CAD build for the part. Positions are in the model's coordinates, mm. A direction names the side the tool comes from. Coordinates: 2 decimals unless noted, no trailing zeros. Order: outer loops, then holes, each group sorted by start corner. A loop starts at its lowest first (then second) coordinate and runs counter-clockwise, first axis right, second up. Notation, with made-up numbers: (-32, -34.75) - (-9, -34.75) arc R26 ccw to (-9, 2.25) - close; hole circle Ø4 at (-8.75, -36.5). An arc over 180 degrees is marked (long way). Use one line per item in the form item = value.
```python
from build123d import *

# Parameters (mm, degrees)
SKETCH1_R           = 4.75
BOSS_EXTRUDE1_DEPTH = 4
SKETCH2_R           = 9
BOSS_EXTRUDE2_DEPTH = 4
FILLET1_R           = 2
SHELL1_T            = -1
SKETCH4_R           = 3.75
BOSS_EXTRUDE4_DEPTH = 2


with BuildPart() as part:
    # Sketch1 → Boss-Extrude1 (new body)
    with BuildSketch(Plane(origin=(0, 0, 0), x_dir=(1, 0, 0), z_dir=(0, 1, 0))):
        with Locations(Location((0, 0, 0), (0, 0, 270))):
            Circle(SKETCH1_R)
    extrude(amount=BOSS_EXTRUDE1_DEPTH)

    # Sketch2 → Boss-Extrude2 (add)
    with BuildSketch(Plane(origin=(0, 4, 0), x_dir=(1, 0, 0), z_dir=(0, 1, 0))):
        with Locations(Location((0, 0, 0), (0, 0, 270))):
            Circle(SKETCH2_R)
    extrude(amount=BOSS_EXTRUDE2_DEPTH)

    # Fillet1
    fillet1_edges = [part.edges().sort_by_distance(p)[0] for p in [
        (0, 4, -9),
        (0, 8, -9),
    ]]
    fillet(fillet1_edges, radius=FILLET1_R - 0.0001)  # a hair under: the kernel refuses the full size

    # Sketch5 → Revolve1 (revolve)
    with BuildSketch(Plane.XY, mode=Mode.PRIVATE) as revolve1_sk:
        with BuildLine():
            Line((0, -7.5), (0, 0.817821063))
            ThreePointArc((0, 0.817821063), (7.716640254, -1.439591085), (13, -7.5))
            Line((13, -7.5), (0, -7.5))
        make_face()
    revolve(revolve1_sk.sketch.rotate(Axis((0, -7.5, 0), (0, 1, 0)), 270), axis=Axis((0, -7.5, 0), (0, 1, 0)))

    # Shell1
    shell1_openings = [part.faces().sort_by_distance(p)[0] for p in [
        (0, -7.5, 0),
    ]]
    offset(amount=SHELL1_T, openings=shell1_openings, kind=Kind.INTERSECTION)

    # Sketch4 → Boss-Extrude4 (add)
    with BuildSketch(Plane(origin=(0, 0, 0), x_dir=(-1, 0, 0), z_dir=(0, -1, 0))):
        with Locations(Location((0, 0, 0), (0, 0, 90))):
            Circle(SKETCH4_R)
    extrude(amount=-BOSS_EXTRUDE4_DEPTH)


solid = part.part
```
Item 1: Cut at D-D, the plane z = -6.5. State how many separate pieces and enclosed holes the cut face has, plus the area to 3 significant figures.
Derived:
separate_pieces = 2
enclosed_holes = 1
area = 56.6 mm²
Item 2: Cut at C-C, the plane y = 2.5. Write the cut outline in (x, z).
Derived:
outline = circle Ø9.5 at (0, 0); hole circle Ø7.5 at (0, 0)
Item 3: Drill centre lines: line 1 (X direction, y = 3.9, z = 0); line 2 (Y direction, x = -7.5, z = 0); line 3 (Y direction, x = 7.75, z = -1.5). Where is each one in solid material? Low to high. Write a range as [from, to].
Derived:
line_1 = [-4.75, -3.75], [3.75, 4.75]
line_2 = [-2.49, -1.3], [4.06, 5.13], [6.87, 7.94]
line_3 = [-2.77, -1.55], [4.21, 5.55], [6.45, 7.79]
Item 4: Two-plate mould, pull along Y, no slides. Class faces 1 (the face through (-11, -7.5, 6)), 2 (the face through (0, 8, 0)), 3 (the face through (-2.89, 1.98, -3.77)): +Y half, -Y half, draft (parallel to the pull), parting line (faces both ways), or undercut.
Derived:
face_1 = -Y half
face_2 = +Y half
face_3 = undercut
Item 5: Drop flat-ended pins along their axis: pin 1 (7 mm diameter, centred on x = 2, z = -0.5, fed in from -Y); pin 2 (7 mm diameter, centred on x = 0, z = 0, fed in from -Y); pin 3 (1.5 mm diameter, centred on y = 1, z = -4.5, fed in from -X). Give the stop position or say it passes through.
Derived:
pin_1 = -1.4
pin_2 = 0
pin_3 = -2.92
Item 6: 3-axis set-ups, long thin cutter, end or side, ignore diameter. For faces 4 (the face through (0.165, -0.366, -3.746)), 5 (the face through (0, 2, 0)): which of +Z, -Z, +X, -X, +Y, -Y reach the whole face in a straight line?
Derived:
face_4 = -Y
face_5 = none
